Here's how the part is built. I have some questions about the finished solid (model axes, mm). Face numbers are marked on the shaded views. A direction names the side the tool comes from. Round coordinates to 2 decimals unless told otherwise and drop trailing zeros. Loops run counter-clockwise (first coordinate to the right, second up) from the corner with the lowest first, then second, coordinate; pieces in that order, holes last. Notation, with made-up numbers: M -20.5,46.25 L 22.5,46.25 A22 ccw 22.5,52.25 Z; hole C 61,17 d1. An arc over 180 degrees is marked long. Use a Markdown table: item, result.
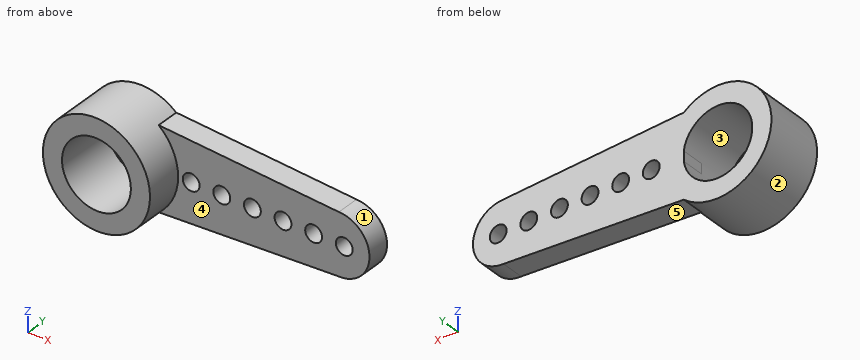
```python
from build123d import *

# Parameters (mm, degrees)
SKETCH1_R           = 3.5
SKETCH1_R_2         = 2.25
BOSS_EXTRUDE1_DEPTH = 3.9
SKETCH2_R           = 2
BOSS_EXTRUDE2_DEPTH = 1.5
SKETCH3_R           = 0.55
CUT_EXTRUDE1_DEPTH  = 1.5
LPATTERN1_COUNT     = 6
LPATTERN1_PITCH     = 2


with BuildPart() as part:
    # Sketch1 → Boss-Extrude1 (new body)
    with BuildSketch(Plane(origin=(0, 0, 0), x_dir=(1, 0, 0), z_dir=(0, 1, 0))):
        Circle(SKETCH1_R)
        Circle(SKETCH1_R_2, mode=Mode.SUBTRACT)
    extrude(amount=-BOSS_EXTRUDE1_DEPTH)

    # Sketch2 → Boss-Extrude2 (add)
    with BuildSketch(Plane(origin=(0, 0, 0), x_dir=(1, 0, 0), z_dir=(0, 1, 0))):
        with BuildLine():
            ThreePointArc((14, -2), (12, 0), (14, 2))
            Line((14, 2), (2.227105745, 2.7))
            Line((2.227105745, 2.7), (2.227105745, -2.7))
            Line((2.227105745, -2.7), (14, -2))
        make_face()
        with Locations((14, 0)):
            Circle(SKETCH2_R)
    extrude(amount=-BOSS_EXTRUDE2_DEPTH)

    # Sketch3 → Cut-Extrude1 (cut)
    with BuildSketch(Plane(origin=(0, 0, 0), x_dir=(1, 0, 0), z_dir=(0, 1, 0))):
        with Locations((14.35, 0)):
            Circle(SKETCH3_R)
    cut_extrude1 = extrude(amount=-CUT_EXTRUDE1_DEPTH, mode=Mode.SUBTRACT)

    # LPattern1: Cut-Extrude1 ×6
    with Locations(*[(-i * LPATTERN1_PITCH, 0, 0) for i in range(1, LPATTERN1_COUNT)]):
        add(cut_extrude1, mode=Mode.SUBTRACT)


solid = part.part
```
Q1. We'd pull the mould along X, two halves only. Please class the marked faces 3, 4 and 5: pulls with the +X half, pulls with the -X half, needs draft (parallel to the pull), parting line crosses it, or undercut.
Return value:
| item | result |
|---|---|
| face 3 | undercut |
| face 4 | needs draft |
| face 5 | pulls with the +X half |
Q2. Will these pins go through, and if not, where does the flat tip stop? P1, Ø1.8, axis at x = 6.35, z = 0, coming from the -Y side; P2, Ø1, axis at y = -2, z = 2.5, coming from the -X side.
Return value:
| item | result |
|---|---|
| P1 | stops at y = -1.5 |
| P2 | stops at x = -2.87 |
Q3. Imagine slicing it at A-A, the plane x = 0. Please give me the cut outline in (y, z).
Return value:
| item | result |
|---|---|
| outline | M -3.9,-3.5 L 0,-3.5 L 0,-2.25 L -3.9,-2.25 Z; M -3.9,2.25 L 0,2.25 L 0,3.5 L -3.9,3.5 Z |
Q4. Imagine slicing it at B-B, the plane y = -0.7. Please give me the cut outline in (x, z).
Return value:
| item | result |
|---|---|
| outline | M 2.23,-2.7 L 14,-2 A2 ccw 14,2 L 2.23,2.7 A3.5 ccw long Z; hole M 2.23,-0.32 L 2.23,0.32 A2.25 ccw long Z; hole C 4.35,0 d1.1; hole C 6.35,0 d1.1; hole C 8.35,0 d1.1; hole C 10.35,0 d1.1; hole C 12.35,0 d1.1; hole C 14.35,0 d1.1 |
Q5. I need wall thicknesses on line 1 (Z direction, x = 0, y = -0.85); line 2 (Y direction, x = 5.5, z = -0.25); line 3 (Z direction, x = 4.35, y = -0.75). Which ranges of each line are inside material? Lowest first, please. Write a range as from..to.
Return value:
| item | result |
|---|---|
| line 1 | z = -3.5..-2.25, 2.25..3.5 |
| line 2 | y = -1.5..0 |
| line 3 | z = -2.57..-0.55, 0.55..2.57 |
Q6. Imagine slicing it at C-C, the plane z = 1. Please give me the cut outline in (x, y).
Return value:
| item | result |
|---|---|
| outline | M -3.35,-3.9 L -2.02,-3.9 L -2.02,0 L -3.35,0 Z; M 2.02,-3.9 L 3.35,-3.9 L 3.35,-1.5 L 15.73,-1.5 L 15.73,0 L 2.02,0 Z |
Q7. For the marked faces 1 and 2, which set-ups out of +Z, -Z, +X, -X, +Y, -Y let a thin tool reach every point of the face, with its end or its side?
Return value:
| item | result |
|---|---|
| face 1 | +X, +Y, -Y |
| face 2 | -Y |
Q8. Imagine slicing it at D-D, the plane y = -1.9. Please give me the cut outline in (x, z).
Return value:
| item | result |
|---|---|
| outline | C 0,0 d7; hole C 0,0 d4.5 |
